For this review, take the finished solid that the model builds, in its own axes (mm). A direction names the side the tool comes from. Coordinates: 2 decimals unless noted, no trailing zeros. Order: outer loops, then holes, each group sorted by start corner. A loop starts at its lowest first (then second) coordinate and runs counter-clockwise, first axis right, second up. Notation, with made-up numbers: (33.25, 59.5) -> (52.25, 59.5) arc R22 cw to (52.25, 81.5) -> close; hole circle Ø5 at (40, 36). An arc over 180 degrees is marked (long way). Write item = value, one per line. Start each with the question number.
1) Consider section B-B on y = 282. Give the boundary of the cut face in (x, z), and give its area (3 significant figures).
2) Wall thickness on probe 1 along Y at (x, z) = (-55, 0.5); probe 2 along Y at (x, z) = (132, 251.5); probe 3 along X at (y, z) = (66.5, -42.5): over which ranges is each line inside the solid? List them lowest first. Write a range as [from, to].
3) Machinability: for faces 1 (the face through (-140, 8, 116)), 2 (the face through (-214, 220, 106)), 3 (the face through (244.779, 167, 112)), which of the approach directions +Z, -Z, +X, -X, +Y, -Y give a long, thin tool a straight path to every point of the face, cutting with its end or side? Answer none if there is none.
4) Draft analysis for pull direction X (two halves, no side actions). For faces 4 (the face through (-507.221, 109, 116)), 5 (the face through (-515.221, 108, 112)), 6 (the face through (-137, 213, 313.85)), state which applies: +X half, -X half, draft (parallel to the pull), parting line (faces both ways), or undercut.
5) Insertion check: pin 1 Ø6 at (x, z) = (-212, -15) entering from -Y; pin 2 Ø1.5 at (x, z) = (-396, 43.5) entering from +Y; pin 3 Ø10 at (y, z) = (258, 153) entering from -X; pin 4 Ø1 at (x, y) = (-116.5, 94) entering from +Z. Each pin has a flat end and moves straight along its axis. Give the tip position at first contact, or say it passes through.
6) Consider section C-C on x = -410.5. Give the boundary of the cut face in (y, z), and give its area (3 significant figures).
7) Consider section A-A on z = 70. Give the boundary of the cut face in (x, y), and give its area (3 significant figures).
from build123d import *

# Parameters (mm, degrees)
SKETCH1_W           = 610
SKETCH1_H           = 410
BOSS_EXTRUDE1_DEPTH = 220
SKETCH2_W           = 410
SKETCH2_H           = 330
BOSS_EXTRUDE2_DEPTH = 150
SKETCH3_W           = 602
SKETCH3_H           = 204
CUT_EXTRUDE1_DEPTH  = 402
SKETCH5_W           = 142
SKETCH5_H           = 204
CUT_EXTRUDE2_DEPTH  = 402
SKETCH6_W           = 134
SKETCH6_H           = 110
CUT_EXTRUDE3_DEPTH  = 402


with BuildPart() as part:
    # Sketch1 → Boss-Extrude1 (new body)
    with BuildSketch(Plane(origin=(0, 0, 0), x_dir=(1, 0, 0), z_dir=(0, 1, 0))):
        with Locations((-210.221238938, -108.849557522)):
            Rectangle(SKETCH1_W, SKETCH1_H)
    extrude(amount=BOSS_EXTRUDE1_DEPTH)

    # Sketch2 → Boss-Extrude2 (add)
    with BuildSketch(Plane(origin=(94.778761062, 0, 0), x_dir=(0, 0, -1), z_dir=(1, 0, 0))):
        with Locations((-108.849557522, 165)):
            Rectangle(SKETCH2_W, SKETCH2_H)
    extrude(amount=BOSS_EXTRUDE2_DEPTH)

    # Sketch3 → Cut-Extrude1 (cut)
    with BuildSketch(Plane.XY.offset(313.849557522)):
        with Locations((-206.221238938, 110)):
            Rectangle(SKETCH3_W, SKETCH3_H)
    extrude(amount=-CUT_EXTRUDE1_DEPTH, mode=Mode.SUBTRACT)

    # Sketch5 → Cut-Extrude2 (cut)
    with BuildSketch(Plane.XY.offset(313.849557522)):
        with Locations((165.778761062, 110)):
            Rectangle(SKETCH5_W, SKETCH5_H)
    extrude(amount=-CUT_EXTRUDE2_DEPTH, mode=Mode.SUBTRACT)

    # Sketch6 → Cut-Extrude3 (cut)
    with BuildSketch(Plane.XY.offset(313.849557522)):
        with Locations((169.778761062, 267)):
            Rectangle(SKETCH6_W, SKETCH6_H)
    extrude(amount=-CUT_EXTRUDE3_DEPTH, mode=Mode.SUBTRACT)


solid = part.part
Answer sheet:
q1.outline = (94.78, -96.15) -> (244.78, -96.15) -> (244.78, 313.85) -> (236.78, 313.85) -> (236.78, -88.15) -> (102.78, -88.15) -> (102.78, 313.85) -> (94.78, 313.85) -> close
q1.area = 7,630 mm2
q2.probe_1 = [0, 8], [212, 220]
q2.probe_2 = [0, 8], [322, 330]
q2.probe_3 = [-515.22, -507.22], [236.78, 244.78]
q3.face_1 = +Z
q3.face_2 = +Z, -Z, -X, +Y
q3.face_3 = +Z, -Z, +X, +Y, -Y
q4.face_4 = undercut
q4.face_5 = -X half
q4.face_6 = draft
q5.pin_1 = 0
q5.pin_2 = 220
q5.pin_3 = 94.78
q5.pin_4 = -88.15
q6.outline = (0, -96.15) -> (220, -96.15) -> (220, 313.85) -> (212, 313.85) -> (212, -88.15) -> (8, -88.15) -> (8, 313.85) -> (0, 313.85) -> close
q6.area = 8,190 mm2
q7.outline = (-515.22, 0) -> (244.78, 0) -> (244.78, 330) -> (94.78, 330) -> (94.78, 220) -> (-515.22, 220) -> close; hole (-507.22, 8) -> (236.78, 8) -> (236.78, 322) -> (102.78, 322) -> (102.78, 212) -> (-507.22, 212) -> close
q7.area = 17,200 mm2
